Geometry check sheet. Reference: the model listing, model coordinates, mm. A direction names the side the tool comes from. Give positions to 0.01 mm unless a question says otherwise; leave off trailing zeros. Order: outer loops, then holes, each group sorted by start corner. A loop starts at its lowest first (then second) coordinate and runs counter-clockwise, first axis right, second up.
from build123d import *

# Parameters (mm, degrees)
F0_R     = 29.5
F0_R_2   = 25.5
F1_DEPTH = 25.5
F2_R     = 104.5
F2_R_2   = 29.5
F3_DEPTH = 5


with BuildPart() as f1:
    # F0 (on Front) → F1 (new body, symmetric)
    with BuildSketch(Plane.XZ):
        Circle(F0_R)
        Circle(F0_R_2, mode=Mode.SUBTRACT)
    extrude(amount=F1_DEPTH, both=True)

    # F2 (on face) → F3 (join)
    with BuildSketch(Plane.XZ.offset(25.5)):
        Circle(F2_R)
        Circle(F2_R_2, mode=Mode.SUBTRACT)
    extrude(amount=-F3_DEPTH)

    # F4: F1 across plane


with BuildPart() as f1_1:
    add(f1.part)
    add(f1.part.mirror(Plane.XZ))


solid = f1_1.part
Item 1: Gauge pin test, flat ends, axial feed: pin 1 (10 mm diameter, centred on y = 13.5, z = -67, fed in from -X); pin 2 (12 mm diameter, centred on y = 6, z = -31.5, fed in from +X). Record the tip position at first contact, or that the pin passes through.
Reported:
pin 1: passes through
pin 2: stops at x = 14.83
Item 2: Sectioned sample at B-B (x = 0). Enter the section's corners in (y, z).
Reported:
outline: (-25.5, -104.5) - (-20.5, -104.5) - (-20.5, -29.5) - (20.5, -29.5) - (20.5, -104.5) - (25.5, -104.5) - (25.5, -25.5) - (-25.5, -25.5) - close; (-25.5, 25.5) - (25.5, 25.5) - (25.5, 104.5) - (20.5, 104.5) - (20.5, 29.5) - (-20.5, 29.5) - (-20.5, 104.5) - (-25.5, 104.5) - close
Item 3: Scan lines: L1, parallel to Z at x = 0, y = -3; L2, parallel to Y at x = 61.5, z = 64; L3, parallel to Z at x = 18, y = -5.5. Record each from-to range of solid material in increasing order.
Reported:
L1: z = -29.5 to -25.5, 25.5 to 29.5
L2: y = -25.5 to -20.5, 20.5 to 25.5
L3: z = -23.37 to -18.06, 18.06 to 23.37
Item 4: Sectioned sample at D-D (x = -84). Enter the section's corners in (y, z), and give its area (3 significant figures).
Reported:
outline: (-25.5, -62.16) - (-20.5, -62.16) - (-20.5, 62.16) - (-25.5, 62.16) - close; (20.5, -62.16) - (25.5, -62.16) - (25.5, 62.16) - (20.5, 62.16) - close
area: 1,240 mm2
Item 5: Set-up check for faces 1 (the flat face through (22, 25.5, -22)), 2 (the cylindrical face through (28.14, -0.29, 8.86)): record each of +Z, -Z, +X, -X, +Y, -Y from which the full face is reachable in a straight line by a thin tool's end or side.
Reported:
face 1: +Z, -Z, +X, -X, +Y
face 2: none
Item 6: Draft check along X on faces 3 (the flat face through (22, -25.5, -22)), 4 (the cylindrical face through (56.2, -23, 88.1)), 5 (the cylindrical face through (-5.5, 0.4, -24.9)). Enter one of: released by +X, released by -X, zero draft, split by the parting line, or undercut.
Reported:
face 3: zero draft
face 4: split by the parting line
face 5: undercut
Item 7: Sectioned sample at A-A (z = 0). Enter the section's corners in (x, y), and give its area (3 significant figures).
Reported:
outline: (-104.5, -25.5) - (-25.5, -25.5) - (-25.5, 25.5) - (-104.5, 25.5) - (-104.5, 20.5) - (-29.5, 20.5) - (-29.5, -20.5) - (-104.5, -20.5) - close; (25.5, -25.5) - (104.5, -25.5) - (104.5, -20.5) - (29.5, -20.5) - (29.5, 20.5) - (104.5, 20.5) - (104.5, 25.5) - (25.5, 25.5) - close
area: 1,910 mm2
Item 8: Sectioned sample at C-C (y = 18). Enter the section's corners in (x, z).
Reported:
outline: circle Ø59 at (0, 0); hole circle Ø51 at (0, 0)
